The model under review builds one solid part; all positions refer to its coordinate system, in mm. Round coordinates to 2 decimals unless told otherwise and drop trailing zeros. Write each loop counter-clockwise with the first axis right and the second up, starting at its lowest first coordinate (ties: lowest second). Pieces come first, ordered by that corner, then holes. Notation, with made-up numbers: (10.5, -28) - (37.5, -28) arc R26 ccw to (37.5, 10) - close; hole circle Ø2 at (25, 65). An arc over 180 degrees is marked (long way). Use one line per item in the form item = value.
from build123d import *

# Parameters (mm, degrees)
F0_R     = 5.25
F1_DEPTH = 22.25
F2_R     = 2.5
F3_DEPTH = 1.5
F4_R     = 0.762


with BuildPart() as f1:
    # F0 (on Top) → F1 (new body, symmetric)
    with BuildSketch(Plane.XY):
        Circle(F0_R)
    extrude(amount=F1_DEPTH, both=True)

    # F2 (on face) → F3 (join)
    with BuildSketch(Plane.XY.offset(22.25)):
        Circle(F2_R)
    extrude(amount=F3_DEPTH)

    # F4
    f4_edges = [f1.edges().sort_by_distance(p)[0] for p in [
        (-2.5, 0, 23.75),
        (-5.25, 0, -22.25),
        (-5.25, 0, 22.25),
    ]]
    fillet(f4_edges, radius=F4_R)


solid = f1.part
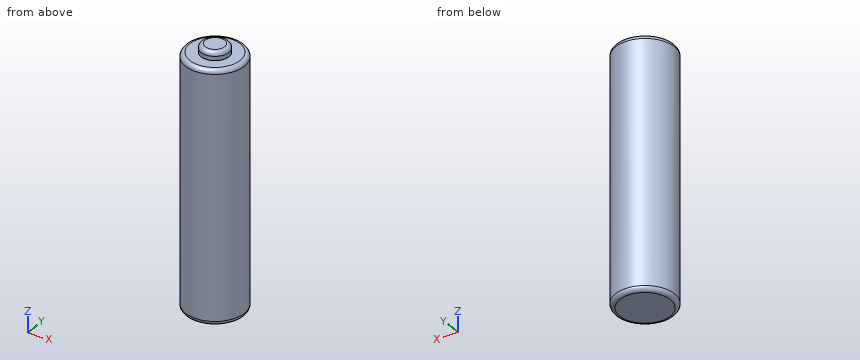
(1) Insertion check: P1, Ø1, axis at x = 2, z = -4.5, coming from the -Y side; P2, Ø4, axis at y = -3, z = -8.5, coming from the +X side; P3, Ø3, axis at x = -2.5, y = -3.5, coming from the +Z side. Each pin has a flat end and moves straight along its axis. Give the tip position at first contact, or say it passes through.
Geometry results:
P1 = -5.03
P2 = 5.15
P3 = 22.25
(2) To check wall thickness, follow L1, parallel to Z at x = 3.5, y = 2.5; L2, parallel to Y at x = -0.25, z = 12.5; L3, parallel to X at y = 0.5, z = 14. State the ranges of each line that lie inside material, in increasing order.
Geometry results:
L1 = -22.25 to 22.25
L2 = -5.24 to 5.24
L3 = -5.23 to 5.23
(3) Add section C-C on z = -5. Write out the cut boundary in (x, y).
Geometry results:
outline = circle Ø10.5 at (0, 0)
(4) Add section A-A on y = 0. Write out the cut boundary in (x, z), then the cut area to 3 significant figures.
Geometry results:
outline = (-5.25, -21.49) arc R0.76 ccw to (-4.49, -22.25) - (4.49, -22.25) arc R0.76 ccw to (5.25, -21.49) - (5.25, 21.49) arc R0.76 ccw to (4.49, 22.25) - (2.5, 22.25) - (2.5, 22.99) arc R0.76 ccw to (1.74, 23.75) - (-1.74, 23.75) arc R0.76 ccw to (-2.5, 22.99) - (-2.5, 22.25) - (-4.49, 22.25) arc R0.76 ccw to (-5.25, 21.49) - close
area = 474 mm2
